from build123d import *

# Parameters (mm, degrees)
EXTRUDE_1_DEPTH          = 2
EXTRUDE_1_2_DEPTH        = 2
EXTRUDE_1_3_DEPTH        = 2
EXTRUDE_1_4_DEPTH        = 2
EXTRUDE_2_DEPTH          = 8
SKETCH_5_R               = 22
SKETCH_5_R_2             = 20.5
EXTRUDE_3_DEPTH          = 8
SKETCH_6_R               = 16.5
SKETCH_6_R_2             = 15.5
EXTRUDE_4_DEPTH          = 7
CUT_EXTRUDE_START        = -10
SKETCH_7_R               = 15.5
CUT_EXTRUDE_1_DEPTH      = 10
SKETCH_8_W               = 15
SKETCH_8_H               = 5
CUT_EXTRUDE_2_DEPTH      = 36.944401511
PATTERN_CIRCULAR_1_COUNT = 2
PATTERN_CIRCULAR_1_ANGLE = 90
EXTRUDE_5_DEPTH          = 2
CUT_EXTRUDE_START_2      = 30
SKETCH_10_R              = 0.5
CUT_EXTRUDE_3_DEPTH      = 10
CUT_EXTRUDE_START_3      = -2
SKETCH_16_R              = 21
CUT_EXTRUDE_5_DEPTH      = 2


with BuildPart() as part:
    # Sketch 1 → Extrude 1 (new body)
    with BuildSketch(Plane(origin=(0, 0, 0), x_dir=(1, 0, 0), z_dir=(0, 1, 0))):
        with BuildLine():
            Line((-10.591663047, 21.536403458), (-10.591663047, 19.282548429))
            ThreePointArc((-10.591663047, 19.282548429), (-15.556349186, 15.556349186), (-19.282548429, 10.591663047))
            Line((-19.282548429, 10.591663047), (-21.536403458, 10.591663047))
            ThreePointArc((-21.536403458, 10.591663047), (-16.970562748, 16.970562748), (-10.591663047, 21.536403458))
        make_face()
    extrude(amount=EXTRUDE_1_DEPTH)



with BuildPart() as body_2:
    # Sketch 1 → Extrude 1 2 (new body)
    with BuildSketch(Plane(origin=(0, 0, 0), x_dir=(1, 0, 0), z_dir=(0, 1, 0))):
        with BuildLine():
            Line((10.591663047, 21.536403458), (10.591663047, 19.282548429))
            ThreePointArc((10.591663047, 19.282548429), (15.556349186, 15.556349186), (19.282548429, 10.591663047))
            Line((19.282548429, 10.591663047), (21.536403458, 10.591663047))
            ThreePointArc((21.536403458, 10.591663047), (16.970562748, 16.970562748), (10.591663047, 21.536403458))
        make_face()
    extrude(amount=EXTRUDE_1_2_DEPTH)


with BuildPart() as body_3:
    # Sketch 1 → Extrude 1 3 (new body)
    with BuildSketch(Plane(origin=(0, 0, 0), x_dir=(1, 0, 0), z_dir=(0, 1, 0))):
        with BuildLine():
            Line((-21.536403458, -10.591663047), (-19.282548429, -10.591663047))
            ThreePointArc((-19.282548429, -10.591663047), (-15.556349186, -15.556349186), (-10.591663047, -19.282548429))
            Line((-10.591663047, -19.282548429), (-10.591663047, -21.536403458))
            ThreePointArc((-10.591663047, -21.536403458), (-16.970562748, -16.970562748), (-21.536403458, -10.591663047))
        make_face()
    extrude(amount=EXTRUDE_1_3_DEPTH)


with BuildPart() as body_4:
    # Sketch 1 → Extrude 1 4 (new body)
    with BuildSketch(Plane(origin=(0, 0, 0), x_dir=(1, 0, 0), z_dir=(0, 1, 0))):
        with BuildLine():
            Line((21.536403458, -10.591663047), (19.282548429, -10.591663047))
            ThreePointArc((19.282548429, -10.591663047), (15.556349186, -15.556349186), (10.591663047, -19.282548429))
            Line((10.591663047, -19.282548429), (10.591663047, -21.536403458))
            ThreePointArc((10.591663047, -21.536403458), (16.970562748, -16.970562748), (21.536403458, -10.591663047))
        make_face()
    extrude(amount=EXTRUDE_1_4_DEPTH)


with BuildPart() as part_1:
    add(part.part)

    add(body_2.part)  # Extrude 2 merges body 2

    add(body_3.part)  # Extrude 2 merges body 3

    add(body_4.part)  # Extrude 2 merges body 4
    # Sketch 4 → Extrude 2 (add)
    with BuildSketch(Plane(origin=(0, 2, 0), x_dir=(1, 0, 0), z_dir=(0, 1, 0))):
        with BuildLine():
            Line((-10.591663047, 21.536403458), (-10.591663047, 19.282548429))
            ThreePointArc((-10.591663047, 19.282548429), (0, 22), (10.591663047, 19.282548429))
            Line((10.591663047, 19.282548429), (10.591663047, 21.536403458))
            ThreePointArc((10.591663047, 21.536403458), (16.970562748, 16.970562748), (21.536403458, 10.591663047))
            Line((21.536403458, 10.591663047), (19.282548429, 10.591663047))
            ThreePointArc((19.282548429, 10.591663047), (22, 0), (19.282548429, -10.591663047))
            Line((19.282548429, -10.591663047), (21.536403458, -10.591663047))
            ThreePointArc((21.536403458, -10.591663047), (16.970562748, -16.970562748), (10.591663047, -21.536403458))
            Line((10.591663047, -21.536403458), (10.591663047, -19.282548429))
            ThreePointArc((10.591663047, -19.282548429), (0, -22), (-10.591663047, -19.282548429))
            Line((-10.591663047, -19.282548429), (-10.591663047, -21.536403458))
            ThreePointArc((-10.591663047, -21.536403458), (-16.970562748, -16.970562748), (-21.536403458, -10.591663047))
            Line((-21.536403458, -10.591663047), (-19.282548429, -10.591663047))
            ThreePointArc((-19.282548429, -10.591663047), (-22, 0), (-19.282548429, 10.591663047))
            Line((-19.282548429, 10.591663047), (-21.536403458, 10.591663047))
            ThreePointArc((-21.536403458, 10.591663047), (-16.970562748, 16.970562748), (-10.591663047, 21.536403458))
        make_face()
    extrude(amount=EXTRUDE_2_DEPTH)

    # Sketch 5 → Extrude 3 (add)
    with BuildSketch(Plane(origin=(0, 10, 0), x_dir=(1, 0, 0), z_dir=(0, 1, 0))):
        with Locations(Location((0, 0, 0), (0, 0, 61.22055739))):
            Circle(SKETCH_5_R)
        with Locations(Location((0, 0, 0), (0, 0, 270))):
            Circle(SKETCH_5_R_2, mode=Mode.SUBTRACT)
    extrude(amount=EXTRUDE_3_DEPTH)

    # Sketch 6 → Extrude 4 (add)
    with BuildSketch(Plane(origin=(0, 10, 0), x_dir=(1, 0, 0), z_dir=(0, 1, 0))):
        with Locations(Location((0, 0, 0), (0, 0, 270))):
            Circle(SKETCH_6_R)
        with Locations(Location((0, 0, 0), (0, 0, 270))):
            Circle(SKETCH_6_R_2, mode=Mode.SUBTRACT)
    extrude(amount=EXTRUDE_4_DEPTH)

    # Sketch 7 → Cut-Extrude 1 (cut)
    with BuildSketch(Plane(origin=(0, 10, 0), x_dir=(1, 0, 0), z_dir=(0, 1, 0)).offset(CUT_EXTRUDE_START)):
        with Locations(Location((0, 0, 0), (0, 0, 270))):
            Circle(SKETCH_7_R)
    extrude(amount=CUT_EXTRUDE_1_DEPTH, mode=Mode.SUBTRACT)

    # Sketch 8 → Cut-Extrude 2 (cut, symmetric)
    with BuildSketch(Plane.XY):
        with Locations((0, 4.5)):
            Rectangle(SKETCH_8_W, SKETCH_8_H)
    cut_extrude_2 = extrude(amount=CUT_EXTRUDE_2_DEPTH, both=True, mode=Mode.SUBTRACT)

    # Pattern Circular 1: Cut-Extrude 2 ×2 about axis
    pattern_circular_1_axis = Axis((0, 10, 0), (0, -1, 0))
    for i in range(1, PATTERN_CIRCULAR_1_COUNT):
        add(cut_extrude_2.rotate(pattern_circular_1_axis, i * PATTERN_CIRCULAR_1_ANGLE / (PATTERN_CIRCULAR_1_COUNT - 1)), mode=Mode.SUBTRACT)

    # Sketch 9 → Extrude 5 (add)
    with BuildSketch(Plane(origin=(0, 18, 0), x_dir=(1, 0, 0), z_dir=(0, 1, 0))):
        with BuildLine():
            Line((1, -20.976176963), (1, -21.977260976))
            ThreePointArc((1, -21.977260976), (22, 0), (1, 21.977260976))
            Line((1, 21.977260976), (1, 20.976176963))
            ThreePointArc((1, 20.976176963), (21, 0), (1, -20.976176963))
        make_face()
        with BuildLine():
            Line((-1, 20.976176963), (-1, 21.977260976))
            ThreePointArc((-1, 21.977260976), (-22, 0), (-1, -21.977260976))
            Line((-1, -21.977260976), (-1, -20.976176963))
            ThreePointArc((-1, -20.976176963), (-21, 0), (-1, 20.976176963))
        make_face()
    extrude(amount=EXTRUDE_5_DEPTH)

    # Sketch 10 → Cut-Extrude 3 (cut)
    with BuildSketch(Plane.XY.offset(CUT_EXTRUDE_START_2)):
        with Locations((-2, 13)):
            Circle(SKETCH_10_R)
        with Locations((2, 13)):
            Circle(SKETCH_10_R)
    extrude(amount=-CUT_EXTRUDE_3_DEPTH, mode=Mode.SUBTRACT)

    # Sketch 16 → Cut-Extrude 5 (cut)
    with BuildSketch(Plane(origin=(0, 18, 0), x_dir=(1, 0, 0), z_dir=(0, 1, 0)).offset(CUT_EXTRUDE_START_3)):
        with Locations(Location((0, 0, 0), (0, 0, 92.729402637))):
            Circle(SKETCH_16_R)
    extrude(amount=CUT_EXTRUDE_5_DEPTH, mode=Mode.SUBTRACT)


solid = part_1.part
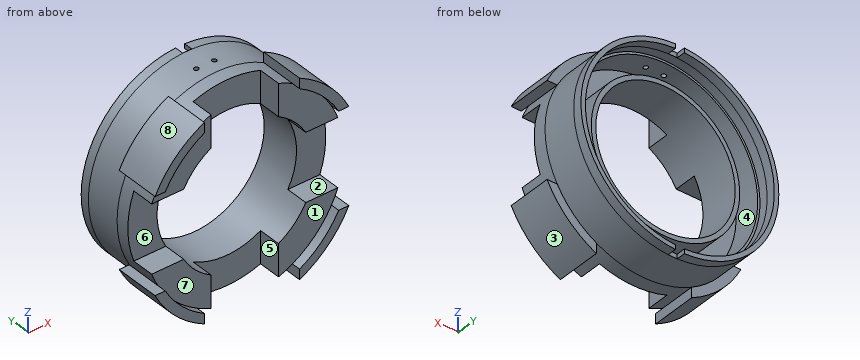
Can you work these out from the model? Positions are in its coordinate system, mm. Face numbers are marked on the shaded views. A direction names the side the tool comes from. Give positions to 0.01 mm unless a question says otherwise; leave off trailing zeros. Order: outer loops, then holes, each group sorted by start corner. A loop starts at its lowest first (then second) coordinate and runs counter-clockwise, first axis right, second up. Notation, with made-up numbers: M 14.25,79.25 L 70.25,79.25 A24 cw 70.25,107.25 Z; hole C -34.5,-0.5 d10. An arc over 180 degrees is marked long. Use one line per item in the form item = value. Start each with the question number.
Item 1: If we section it at A-A (y = 4): State how many separate pieces and enclosed holes the cut face has, then the cut area to 3 significant figures.
Item 2: We'd pull the mould along X, two halves only. Please class the marked faces 6, 7 and 8: +X half, -X half, draft (parallel to the pull), parting line (faces both ways), or undercut.
Item 3: If we section it at C-C (x = 0): Write out the boundary of the cut face in (y, z).
Item 4: If I drill on line 1 along Z through (x, y) = (0, 13.75); line 2 along Z through (x, y) = (0, 16.95), over which ranges is the centre line in solid material (lowest first)?
Item 5: If we section it at D-D (y = 9.25): Write out the boundary of the cut face in (x, z), then the cut area to 3 significant figures.
Item 6: If we section it at B-B (z = 0): Write out the boundary of the cut face in (x, y), then the cut area to 3 significant figures.
Item 7: For the marked faces 1, 2, 3, 4 and 5, which set-ups out of +Z, -Z, +X, -X, +Y, -Y let a thin tool reach every point of the face, with its end or its side?
Item 8: Will these pins go through, and if not, where does the flat tip stop? pin 1 Ø1.8 at (x, y) = (-20.5, 6.5) entering from -Z; pin 2 Ø0.7 at (x, y) = (20.5, 4) entering from +Z; pin 3 Ø3 at (y, z) = (11.5, 2) entering from +X; pin 4 Ø8 at (x, z) = (-7, 3.5) entering from +Y.
Outcome:
q1.separate_pieces = 4
q1.enclosed_holes = 0
q1.area = 477 mm2
q2.face_6 = draft
q2.face_7 = undercut
q2.face_8 = -X half
q3.outline = M 7,-22 L 18,-22 L 18,-21 L 16,-21 L 16,-20.5 L 10,-20.5 L 10,-16.5 L 16,-16.5 L 16,-15.5 L 7,-15.5 Z; M 7,15.5 L 16,15.5 L 16,16.5 L 10,16.5 L 10,20.5 L 16,20.5 L 16,21 L 18,21 L 18,22 L 7,22 Z
q4.line_1 = -22 to -20.5, -16.5 to -15.5, 15.5 to 16.5, 20.5 to 22
q4.line_2 = -22 to -21, 21 to 22
q5.outline = M -21.54,-10.59 A24 ccw -10.59,-21.54 L -10.59,-19.28 A22 ccw 10.59,-19.28 L 10.59,-21.54 A24 ccw 21.54,-10.59 L 19.28,-10.59 A22 ccw 19.28,10.59 L 21.54,10.59 A24 ccw 10.59,21.54 L 10.59,19.28 A22 ccw -10.59,19.28 L -10.59,21.54 A24 ccw -21.54,10.59 L -19.28,10.59 A22 ccw -19.28,-10.59 Z; hole C 0,0 d31
q5.area = 879 mm2
q6.outline = M -22,7 L -15.5,7 L -15.5,16 L -16.5,16 L -16.5,10 L -20.5,10 L -20.5,16 L -21,16 L -21,20 L -22,20 Z; M 15.5,7 L 22,7 L 22,20 L 21,20 L 21,16 L 20.5,16 L 20.5,10 L 16.5,10 L 16.5,16 L 15.5,16 Z
q6.area = 77.0 mm2
q7.face_1 = -Y
q7.face_2 = +X, -X, -Y
q7.face_3 = -Z, +X, +Y, -Y
q7.face_4 = +Y
q7.face_5 = +Z, -Z, -Y
q8.pin_1 = -13.85
q8.pin_2 = 13.04
q8.pin_3 = 21.99
q8.pin_4 = through
